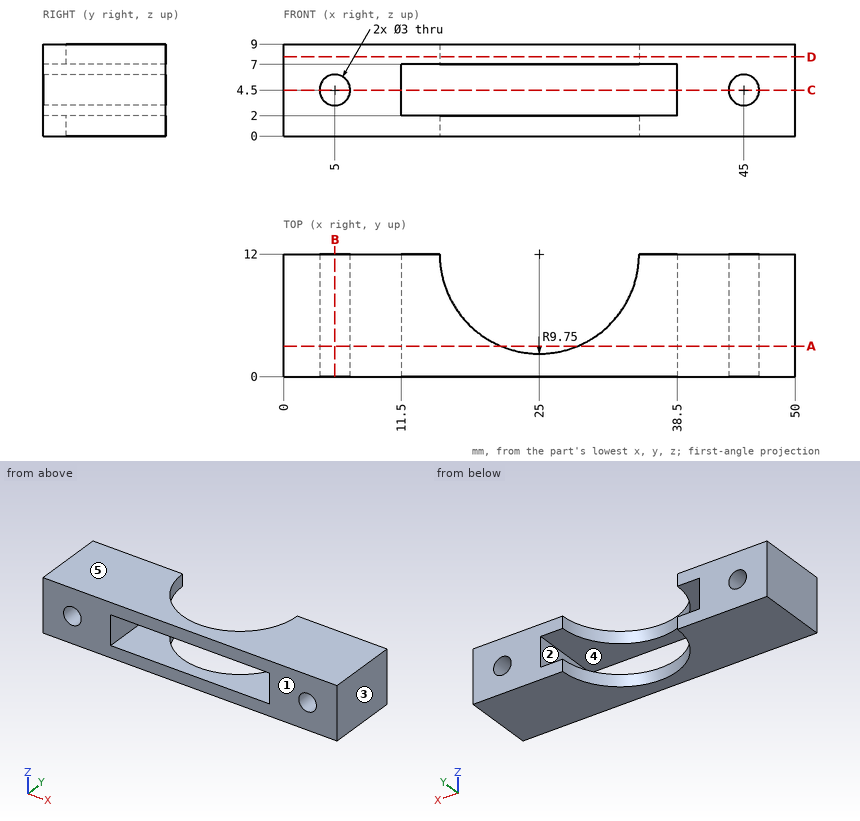
Job drawing, mm, ordinate dimensions from the low corner. One solid piece. A direction names the side the tool comes from. Give positions to 0.01 mm unless a question says otherwise; leave off trailing zeros. Loops run counter-clockwise (first coordinate to the right, second up) from the corner with the lowest first, then second, coordinate; pieces in that order, holes last. Notation, with made-up numbers: (-6, 69.25) -> (41, 69.25) arc R27 ccw to (41, 108.25) -> close; hole circle Ø10 at (-6, -8). An arc over 180 degrees is marked (long way). Write each question's results on one line, items separated by ' | '.
(1) Flat gauge pin, fed straight in: pin 1 Ø1.8 at (x, z) = (45, 4.5) entering from +Y. Where does the tip first touch, or does it go through?
Geometry results:
pin 1: passes through
(2) Probe line 1 along Z through (x, y) = (5, 8); line 2 along X through (y, z) = (3.25, 2.25); line 3 along X through (y, z) = (1, 5). List the from-to ranges inside material, lowest first.
Geometry results:
line 1: z = 0 to 3, 6 to 9 | line 2: x = 0 to 11.5, 38.5 to 50 | line 3: x = 0 to 3.59, 6.41 to 11.5, 38.5 to 43.59, 46.41 to 50
(3) Cut at B-B on x = 5. List the corners of the cut face in (y, z), and give its area (3 significant figures).
Geometry results:
outline: (0, 0) -> (12, 0) -> (12, 3) -> (0, 3) -> close; (0, 6) -> (12, 6) -> (12, 9) -> (0, 9) -> close | area: 72.0 mm²
(4) Cut at A-A on y = 3. List the corners of the cut face in (x, z).
Geometry results:
outline: (0, 0) -> (21.25, 0) -> (21.25, 2) -> (11.5, 2) -> (11.5, 7) -> (21.25, 7) -> (21.25, 9) -> (0, 9) -> close; (28.75, 0) -> (50, 0) -> (50, 9) -> (28.75, 9) -> (28.75, 7) -> (38.5, 7) -> (38.5, 2) -> (28.75, 2) -> close; hole circle Ø3 at (5, 4.5); hole circle Ø3 at (45, 4.5)
(5) Tool access for the marked faces 1 and 2: list every direction of +Z, -Z, +X, -X, +Y, -Y with a clear straight run to the whole face (end or side of a thin tool).
Geometry results:
face 1: +Z, -Z, +X, -X, -Y | face 2: +Y, -Y
(6) Pull direction Z, two halves, no side cores. Call the marked faces 3, 4 and 5: released by +Z, released by -Z, zero draft, split by the parting line, or undercut.
Geometry results:
face 3: zero draft | face 4: undercut | face 5: released by +Z
(7) Cut at C-C on z = 4.5. List the corners of the cut face in (x, y).
Geometry results:
outline: (0, 0) -> (3.5, 0) -> (3.5, 12) -> (0, 12) -> close; (6.5, 0) -> (11.5, 0) -> (11.5, 12) -> (6.5, 12) -> close; (38.5, 0) -> (43.5, 0) -> (43.5, 12) -> (38.5, 12) -> close; (46.5, 0) -> (50, 0) -> (50, 12) -> (46.5, 12) -> close
(8) Cut at D-D on z = 7.75. List the corners of the cut face in (x, y), and give its area (3 significant figures).
Geometry results:
outline: (0, 0) -> (50, 0) -> (50, 12) -> (34.75, 12) arc R9.75 cw to (15.25, 12) -> (0, 12) -> close | area: 451 mm²
